Part model, mm, in its own coordinate system. A direction names the side the tool comes from. Give positions to 0.01 mm unless a question says otherwise; leave off trailing zeros. Loops run counter-clockwise (first coordinate to the right, second up) from the corner with the lowest first, then second, coordinate; pieces in that order, holes last. Notation, with made-up numbers: (76.25, 89.25) -> (132.25, 89.25) arc R20 cw to (132.25, 106.25) -> close; hole circle Ø6 at (-38.5, 46.25). An arc over 180 degrees is marked (long way). Write item = value, one per line.
from build123d import *

# Parameters (mm, degrees)
CROQUIS1_W                          = 114
CROQUIS1_H                          = 114
SALIENTE_EXTRUIR1_DEPTH             = 30
REDONDEO1_R                         = 4
CROQUIS2_W                          = 105
CROQUIS2_H                          = 100
CORTAR_EXTRUIR1_DEPTH               = 27
CROQUIS3_W                          = 105
CROQUIS3_H                          = 12
CORTAR_EXTRUIR2_DEPTH               = 7
CROQUIS5_W                          = 2.5
CROQUIS5_H                          = 1.5
SALIENTE_EXTRUIR2_DEPTH             = 107
SALIENTE_EXTRUIR3_REACH             = 59
SALIENTE_EXTRUIR3_DIRECTION_2_REACH = 59
CROQUIS7_R                          = 0.75
CORTAR_EXTRUIR3_DEPTH               = 4.5


with BuildPart() as part:
    # Croquis1 → Saliente-Extruir1 (new body)
    with BuildSketch(Plane(origin=(0, 0, 0), x_dir=(1, 0, 0), z_dir=(0, 1, 0))):
        Rectangle(CROQUIS1_W, CROQUIS1_H)
    extrude(amount=SALIENTE_EXTRUIR1_DEPTH)

    # Redondeo1
    redondeo1_edges = [part.edges().sort_by_distance(p)[0] for p in [
        (57, 15, 57),
        (-57, 15, 57),
        (-57, 15, -57),
        (57, 15, -57),
    ]]
    fillet(redondeo1_edges, radius=REDONDEO1_R)

    # Croquis2 → Cortar-Extruir1 (cut)
    with BuildSketch(Plane(origin=(0, 30, 0), x_dir=(1, 0, 0), z_dir=(0, 1, 0))):
        Rectangle(CROQUIS2_W, CROQUIS2_H)
    extrude(amount=-CORTAR_EXTRUIR1_DEPTH, mode=Mode.SUBTRACT)

    # Croquis3 → Cortar-Extruir2 (cut)
    with BuildSketch(Plane.XY.offset(57)):
        with Locations((0, 24)):
            Rectangle(CROQUIS3_W, CROQUIS3_H)
    extrude(amount=-CORTAR_EXTRUIR2_DEPTH, mode=Mode.SUBTRACT)

    # Croquis5 → Saliente-Extruir2 (add)
    with BuildSketch(Plane.XY.offset(57)):
        with Locations((-51.25, 20.75)):
            Rectangle(CROQUIS5_W, CROQUIS5_H)
        with Locations((-51.25, 24.25)):
            Rectangle(CROQUIS5_W, CROQUIS5_H)
        with Locations((51.25, 20.75)):
            Rectangle(CROQUIS5_W, CROQUIS5_H)
        with Locations((51.25, 24.25)):
            Rectangle(CROQUIS5_W, CROQUIS5_H)
    extrude(amount=-SALIENTE_EXTRUIR2_DEPTH)

    # Saliente-Extruir3: up to this face of the body (flat: up to its plane)
    saliente_extruir3_end = Plane(part.part.faces().sort_by_distance((0, 16.468085106, -50))[0])
    # Croquis6 → Saliente-Extruir3 (add, up to the picked face)
    with BuildSketch(Plane.XY, mode=Mode.PRIVATE) as saliente_extruir3_sk1:
        Polygon((-52.5, 3), (52.5, 12.18630967), (52.5, 3), align=None)
    saliente_extruir3_tool1 = split(extrude(saliente_extruir3_sk1.sketch, amount=-SALIENTE_EXTRUIR3_REACH, mode=Mode.PRIVATE), bisect_by=saliente_extruir3_end, keep=Keep.BOTH, mode=Mode.PRIVATE)
    add(saliente_extruir3_tool1.solids().sort_by_distance((17.5, 6.062103, 0))[0])

    # Saliente-Extruir3 direction 2: up to this face of the body (flat: up to its plane)
    saliente_extruir3_direction_2_end = Plane(part.part.faces().sort_by_distance((0, 10.5, 50))[0])
    # Croquis6 → Saliente-Extruir3 direction 2 (add, up to the picked face)
    with BuildSketch(Plane.XY, mode=Mode.PRIVATE) as saliente_extruir3_direction_2_sk1:
        Polygon((-52.5, 3), (52.5, 12.18630967), (52.5, 3), align=None)
    saliente_extruir3_direction_2_tool1 = split(extrude(saliente_extruir3_direction_2_sk1.sketch, amount=SALIENTE_EXTRUIR3_DIRECTION_2_REACH, mode=Mode.PRIVATE), bisect_by=saliente_extruir3_direction_2_end, keep=Keep.BOTH, mode=Mode.PRIVATE)
    add(saliente_extruir3_direction_2_tool1.solids().sort_by_distance((17.5, 6.062103, 0))[0])

    # Croquis7 → Cortar-Extruir3 (cut)
    with BuildSketch(Plane.ZY.offset(57)):
        with Locations((0, 3.75)):
            Circle(CROQUIS7_R)
    extrude(amount=-CORTAR_EXTRUIR3_DEPTH, mode=Mode.SUBTRACT)

    # Croquis10 → Revolución1 (revolve)
    with BuildSketch(Plane.XY):
        Polygon((-57, 3), (-62, 3), (-62, 2.75), (-59, 2.2), (-59, 2.45), (-57, 2.45), align=None)
    revolve(axis=Axis((-57, 3.75, 0), (1, 0, 0)))


solid = part.part
1) Slice it at B-B, the plane y = 27.25. List the corners of the cut face in (x, z).
Resolved:
outline = (-57, -53) arc R4 ccw to (-53, -57) -> (53, -57) arc R4 ccw to (57, -53) -> (57, 53) arc R4 ccw to (53, 57) -> (52.5, 57) -> (52.5, -50) -> (-52.5, -50) -> (-52.5, 57) -> (-53, 57) arc R4 ccw to (-57, 53) -> close
2) Drop flat-ended pins along their axis: P1, Ø6.5, axis at y = 16.5, z = -17.5, coming from the -X side; P2, Ø1.5, axis at x = -31, z = 42, coming from the +Y side; P3, Ø4, axis at x = -0.5, y = 20.5, coming from the +Z side. Give the stop position or say it passes through.
Resolved:
P1 = -57
P2 = 4.95
P3 = -50
3) Pull direction X, two halves, no side cores. Call faces 1 (the face through (-4, 30, -51)), 2 (the face through (-1, 18, 54)), 3 (the face through (-55.859, 15.21, 55.797)), 4 (the face through (57, 15, 1)): pulls with the +X half, pulls with the -X half, needs draft (parallel to the pull), parting line crosses it, or undercut.
Resolved:
face_1 = needs draft
face_2 = undercut
face_3 = pulls with the -X half
face_4 = pulls with the +X half
4) Drill centre lines: line 1 along X through (y, z) = (24.25, 12.5); line 2 along X through (y, z) = (22.25, -8); line 3 along Y through (x, z) = (-53.65, 0). Where is each one in solid material? Low to high. Write a range as [from, to].
Resolved:
line_1 = [-57, -50], [50, 57]
line_2 = [-57, -52.5], [52.5, 57]
line_3 = [0, 3], [4.5, 30]
5) Slice it at A-A, the plane z = 47.5. List the corners of the cut face in (x, y), and give its area (3 significant figures).
Resolved:
outline = (-57, 0) -> (57, 0) -> (57, 30) -> (52.5, 30) -> (52.5, 25) -> (50, 25) -> (50, 23.5) -> (52.5, 23.5) -> (52.5, 21.5) -> (50, 21.5) -> (50, 20) -> (52.5, 20) -> (52.5, 12.19) -> (-52.5, 3) -> (-52.5, 20) -> (-50, 20) -> (-50, 21.5) -> (-52.5, 21.5) -> (-52.5, 23.5) -> (-50, 23.5) -> (-50, 25) -> (-52.5, 25) -> (-52.5, 30) -> (-57, 30) -> close
area = 1,080 mm²
6) Which spindle directions (+Z, -Z, +X, -X, +Y, -Y) get a long thin tool onto all of the face, cutting with end or side? Do faces 5 (the face through (-60.81, 4.65, -0.82)), 6 (the face through (52.5, 16, 4)), 7 (the face through (-52.5, 28, 4)). Say none if no direction does.
Resolved:
face_5 = -X
face_6 = none
face_7 = +Z, +Y
7) Slice it at C-C, the plane x = -23. List the corners of the cut face in (y, z), and give its area (3 significant figures).
Resolved:
outline = (0, -57) -> (30, -57) -> (30, -50) -> (5.58, -50) -> (5.58, 50) -> (18, 50) -> (18, 57) -> (0, 57) -> close
area = 894 mm²
